Work out the finished part from the listing and answer in its coordinate system (mm). Face numbers are marked on the shaded views. A direction names the side the tool comes from. Round coordinates to 2 decimals unless told otherwise and drop trailing zeros. Write each loop counter-clockwise with the first axis right and the second up, starting at its lowest first coordinate (ties: lowest second). Pieces come first, ordered by that corner, then holes. Notation, with made-up numbers: (10, 52.5) -> (52, 52.5) arc R21 cw to (52, 60.5) -> close; hole circle Ø5 at (53, -33.75). An arc over 180 degrees is marked (long way). Answer as a JSON object with one key per item and string values. Group by question number.
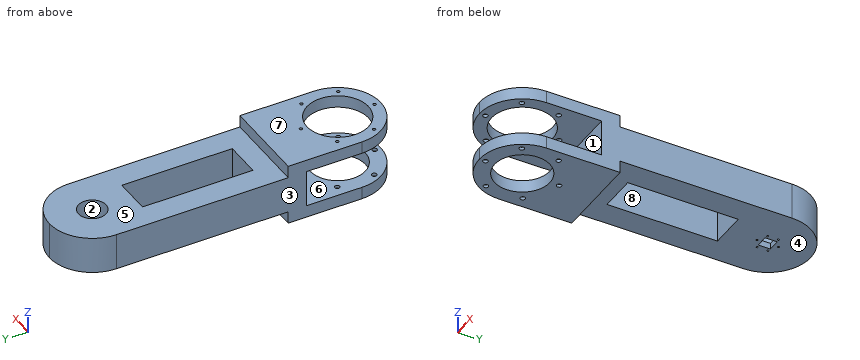
from build123d import *

# Parameters (mm, degrees)
SKETCH_1_W           = 140
SKETCH_1_H           = 350
EXTRUDE_1_DEPTH      = 60
CUT_EXTRUDE_1_REACH  = 199.8
SKETCH_4_W           = 140
SKETCH_4_H           = 100
EXTRUDE_3_DEPTH      = 30
SKETCH_5_W           = 140
SKETCH_5_H           = 20
EXTRUDE_4_DEPTH      = 160
CUT_EXTRUDE_3_DEPTH  = 385.870107959
SKETCH_8_W           = 60
SKETCH_8_H           = 180
CUT_EXTRUDE_4_DEPTH  = 381.164438105
CUT_EXTRUDE_5_REACH  = 386.87
SKETCH_9_R           = 45
CUT_EXTRUDE_6_REACH  = 386.87
SKETCH_10_R          = 50
SKETCH_11_W          = 20
SKETCH_11_H          = 20
CUT_EXTRUDE_7_DEPTH  = 381.164438105
CUT_EXTRUDE_10_REACH = 386.87
SKETCH_13_R          = 2.5
SKETCH_14_R          = 4
CUT_EXTRUDE_11_DEPTH = 5
SKETCH_16_R          = 22.5
SKETCH_16_W          = 20
SKETCH_16_H          = 20
CUT_EXTRUDE_12_DEPTH = 50
SKETCH_17_R          = 1.5
CUT_EXTRUDE_13_DEPTH = 379.186461947
SKETCH_18_R          = 4
CUT_EXTRUDE_14_DEPTH = 5
SKETCH_19_R          = 2.5
CUT_EXTRUDE_15_DEPTH = 385.870107959
CUT_EXTRUDE_START    = -5
SKETCH_20_R          = 4
CUT_EXTRUDE_16_DEPTH = 5


with BuildPart() as part:
    # 草图1 → 凸台-拉伸1 (new body)
    with BuildSketch(Plane.XY):
        Rectangle(SKETCH_1_W, SKETCH_1_H)
    extrude(amount=EXTRUDE_1_DEPTH)

    # 草图2 → 切除-拉伸1 (cut, up to next)
    with BuildSketch(Plane.XY.offset(60), mode=Mode.PRIVATE) as cut_extrude_1_sk1:
        with BuildLine():
            Line((-1.55e-07, 175), (-70, 175))
            Line((-70, 175), (-70, 105))
            ThreePointArc((-70, 105), (-49.497474738, 154.497474628), (-1.55e-07, 175))
        make_face()
    cut_extrude_1_tool1 = extrude(cut_extrude_1_sk1.sketch, amount=-CUT_EXTRUDE_1_REACH, mode=Mode.PRIVATE) & part.part
    # 草图2 → 切除-拉伸1 (cut, up to next)
    with BuildSketch(Plane.XY.offset(60), mode=Mode.PRIVATE) as cut_extrude_1_sk2:
        with BuildLine():
            Line((70, 175), (-1.55e-07, 175))
            ThreePointArc((-1.55e-07, 175), (49.497474628, 154.497474738), (70, 105))
            Line((70, 105), (70, 175))
        make_face()
    cut_extrude_1_tool2 = extrude(cut_extrude_1_sk2.sketch, amount=-CUT_EXTRUDE_1_REACH, mode=Mode.PRIVATE) & part.part
    add(cut_extrude_1_tool1.solids().sort_by_distance((-54.364244, 159.364244, 60))[0], mode=Mode.SUBTRACT)
    add(cut_extrude_1_tool2.solids().sort_by_distance((54.364244, 159.364244, 60))[0], mode=Mode.SUBTRACT)

    # 草图4 → 凸台-拉伸3 (add)
    with BuildSketch(Plane.XZ.offset(175)):
        with Locations((0, 30)):
            Rectangle(SKETCH_4_W, SKETCH_4_H)
    extrude(amount=EXTRUDE_3_DEPTH)

    # 草图5 → 凸台-拉伸4 (add)
    with BuildSketch(Plane.XZ.offset(205)):
        with Locations((0, 70)):
            Rectangle(SKETCH_5_W, SKETCH_5_H)
        with Locations((0, -10)):
            Rectangle(SKETCH_5_W, SKETCH_5_H)
    extrude(amount=EXTRUDE_4_DEPTH)

    # 草图7 → 切除-拉伸3 (cut, through all)
    with BuildSketch(Plane(origin=(0, 0, -20), x_dir=(-1, 0, 0), z_dir=(0, 0, -1))):
        with BuildLine():
            Line((-70, -295), (-70, -365))
            Line((-70, -365), (0, -365))
            ThreePointArc((0, -365), (-49.497474683, -344.497474683), (-70, -295))
        make_face()
        with BuildLine():
            ThreePointArc((70, -295), (49.497474683, -344.497474683), (0, -365))
            Line((0, -365), (70, -365))
            Line((70, -365), (70, -295))
        make_face()
    extrude(amount=-CUT_EXTRUDE_3_DEPTH, mode=Mode.SUBTRACT)

    # 草图8 → 切除-拉伸4 (cut, through all)
    with BuildSketch(Plane(origin=(0, 0, 0), x_dir=(-1, 0, 0), z_dir=(0, 0, -1))):
        with Locations((0, -50)):
            Rectangle(SKETCH_8_W, SKETCH_8_H)
    extrude(amount=-CUT_EXTRUDE_4_DEPTH, mode=Mode.SUBTRACT)

    # 草图9 → 切除-拉伸5 (cut, up to next)
    with BuildSketch(Plane(origin=(0, 0, -20), x_dir=(-1, 0, 0), z_dir=(0, 0, -1)), mode=Mode.PRIVATE) as cut_extrude_5_sk1:
        with Locations((0, -295)):
            Circle(SKETCH_9_R)
    cut_extrude_5_tool1 = extrude(cut_extrude_5_sk1.sketch, amount=-CUT_EXTRUDE_5_REACH, mode=Mode.PRIVATE) & part.part
    add(cut_extrude_5_tool1.solids().sort_by_distance((0, -295, -20))[0], mode=Mode.SUBTRACT)

    # 草图10 → 切除-拉伸6 (cut, up to next)
    with BuildSketch(Plane.XY.offset(80), mode=Mode.PRIVATE) as cut_extrude_6_sk1:
        with Locations((0, -295)):
            Circle(SKETCH_10_R)
    cut_extrude_6_tool1 = extrude(cut_extrude_6_sk1.sketch, amount=-CUT_EXTRUDE_6_REACH, mode=Mode.PRIVATE) & part.part
    add(cut_extrude_6_tool1.solids().sort_by_distance((0, -295, 80))[0], mode=Mode.SUBTRACT)

    # 草图11 → 切除-拉伸7 (cut, through all)
    with BuildSketch(Plane.XY.offset(60)):
        with Locations((0, 105)):
            Rectangle(SKETCH_11_W, SKETCH_11_H)
    extrude(amount=-CUT_EXTRUDE_7_DEPTH, mode=Mode.SUBTRACT)

    # 草图13 → 切除-拉伸10 (cut, up to next)
    with BuildSketch(Plane.XY.offset(80), mode=Mode.PRIVATE) as cut_extrude_10_sk1:
        with Locations((-51.961524227, -265)):
            Circle(SKETCH_13_R)
    cut_extrude_10_tool1 = extrude(cut_extrude_10_sk1.sketch, amount=-CUT_EXTRUDE_10_REACH, mode=Mode.PRIVATE) & part.part
    # 草图13 → 切除-拉伸10 (cut, up to next)
    with BuildSketch(Plane.XY.offset(80), mode=Mode.PRIVATE) as cut_extrude_10_sk2:
        with Locations((0, -235)):
            Circle(SKETCH_13_R)
    cut_extrude_10_tool2 = extrude(cut_extrude_10_sk2.sketch, amount=-CUT_EXTRUDE_10_REACH, mode=Mode.PRIVATE) & part.part
    # 草图13 → 切除-拉伸10 (cut, up to next)
    with BuildSketch(Plane.XY.offset(80), mode=Mode.PRIVATE) as cut_extrude_10_sk3:
        with Locations((51.961524227, -265)):
            Circle(SKETCH_13_R)
    cut_extrude_10_tool3 = extrude(cut_extrude_10_sk3.sketch, amount=-CUT_EXTRUDE_10_REACH, mode=Mode.PRIVATE) & part.part
    # 草图13 → 切除-拉伸10 (cut, up to next)
    with BuildSketch(Plane.XY.offset(80), mode=Mode.PRIVATE) as cut_extrude_10_sk4:
        with Locations((51.961524227, -325)):
            Circle(SKETCH_13_R)
    cut_extrude_10_tool4 = extrude(cut_extrude_10_sk4.sketch, amount=-CUT_EXTRUDE_10_REACH, mode=Mode.PRIVATE) & part.part
    # 草图13 → 切除-拉伸10 (cut, up to next)
    with BuildSketch(Plane.XY.offset(80), mode=Mode.PRIVATE) as cut_extrude_10_sk5:
        with Locations((0, -355)):
            Circle(SKETCH_13_R)
    cut_extrude_10_tool5 = extrude(cut_extrude_10_sk5.sketch, amount=-CUT_EXTRUDE_10_REACH, mode=Mode.PRIVATE) & part.part
    # 草图13 → 切除-拉伸10 (cut, up to next)
    with BuildSketch(Plane.XY.offset(80), mode=Mode.PRIVATE) as cut_extrude_10_sk6:
        with Locations((-51.961524227, -325)):
            Circle(SKETCH_13_R)
    cut_extrude_10_tool6 = extrude(cut_extrude_10_sk6.sketch, amount=-CUT_EXTRUDE_10_REACH, mode=Mode.PRIVATE) & part.part
    add(cut_extrude_10_tool1.solids().sort_by_distance((-51.961524, -265, 80))[0], mode=Mode.SUBTRACT)
    add(cut_extrude_10_tool2.solids().sort_by_distance((0, -235, 80))[0], mode=Mode.SUBTRACT)
    add(cut_extrude_10_tool3.solids().sort_by_distance((51.961524, -265, 80))[0], mode=Mode.SUBTRACT)
    add(cut_extrude_10_tool4.solids().sort_by_distance((51.961524, -325, 80))[0], mode=Mode.SUBTRACT)
    add(cut_extrude_10_tool5.solids().sort_by_distance((0, -355, 80))[0], mode=Mode.SUBTRACT)
    add(cut_extrude_10_tool6.solids().sort_by_distance((-51.961524, -325, 80))[0], mode=Mode.SUBTRACT)

    # 草图14 → 切除-拉伸11 (cut)
    with BuildSketch(Plane(origin=(0, 0, 60), x_dir=(-1, 0, 0), z_dir=(0, 0, -1))):
        with Locations((-51.961524227, -325)):
            Circle(SKETCH_14_R)
        with Locations((-51.961524227, -265)):
            Circle(SKETCH_14_R)
        with Locations((0, -235)):
            Circle(SKETCH_14_R)
        with Locations((51.961524227, -265)):
            Circle(SKETCH_14_R)
        with Locations((51.961524227, -325)):
            Circle(SKETCH_14_R)
        with Locations((0, -355)):
            Circle(SKETCH_14_R)
    extrude(amount=-CUT_EXTRUDE_11_DEPTH, mode=Mode.SUBTRACT)

    # 草图16 → 切除-拉伸12 (cut)
    with BuildSketch(Plane.XY.offset(60)):
        with Locations((0, 105)):
            Circle(SKETCH_16_R)
        with Locations((0, 105)):
            Rectangle(SKETCH_16_W, SKETCH_16_H, mode=Mode.SUBTRACT)
    extrude(amount=-CUT_EXTRUDE_12_DEPTH, mode=Mode.SUBTRACT)

    # 草图17 → 切除-拉伸13 (cut, through all)
    with BuildSketch(Plane.XY.offset(10)):
        with Locations((0, 122.5)):
            Circle(SKETCH_17_R)
        with Locations((15.155444566, 113.75)):
            Circle(SKETCH_17_R)
        with Locations((15.155444566, 96.25)):
            Circle(SKETCH_17_R)
        with Locations((0, 87.5)):
            Circle(SKETCH_17_R)
        with Locations((-15.155444566, 96.25)):
            Circle(SKETCH_17_R)
        with Locations((-15.155444566, 113.75)):
            Circle(SKETCH_17_R)
    extrude(amount=-CUT_EXTRUDE_13_DEPTH, mode=Mode.SUBTRACT)

    # 草图18 → 切除-拉伸14 (cut)
    with BuildSketch(Plane(origin=(0, 0, -20), x_dir=(-1, 0, 0), z_dir=(0, 0, -1))):
        with Locations((0, -235)):
            Circle(SKETCH_18_R)
        with Locations((-51.961524227, -265)):
            Circle(SKETCH_18_R)
        with Locations((-51.961524227, -325)):
            Circle(SKETCH_18_R)
        with Locations((0, -355)):
            Circle(SKETCH_18_R)
        with Locations((51.961524227, -325)):
            Circle(SKETCH_18_R)
        with Locations((51.961524227, -265)):
            Circle(SKETCH_18_R)
    extrude(amount=-CUT_EXTRUDE_14_DEPTH, mode=Mode.SUBTRACT)

    # 草图19 → 切除-拉伸15 (cut, through all)
    with BuildSketch(Plane(origin=(0, 0, -20), x_dir=(-1, 0, 0), z_dir=(0, 0, -1))):
        with Locations(Location((-51.961524227, -265, 0), (0, 0, 180))):
            Circle(SKETCH_19_R)
        with Locations(Location((-51.961524227, -325, 0), (0, 0, 180))):
            Circle(SKETCH_19_R)
        with Locations(Location((0, -355, 0), (0, 0, 180))):
            Circle(SKETCH_19_R)
        with Locations(Location((51.961524227, -325, 0), (0, 0, 180))):
            Circle(SKETCH_19_R)
        with Locations(Location((51.961524227, -265, 0), (0, 0, 180))):
            Circle(SKETCH_19_R)
        with Locations(Location((0, -235, 0), (0, 0, 180))):
            Circle(SKETCH_19_R)
    extrude(amount=-CUT_EXTRUDE_15_DEPTH, mode=Mode.SUBTRACT)

    # 草图20 → 切除-拉伸16 (cut)
    with BuildSketch(Plane.XY.offset(CUT_EXTRUDE_START)):
        with Locations(Location((-51.961524227, -265, 0), (0, 0, 180))):
            Circle(SKETCH_20_R)
        with Locations((0.040572827, -234.996244649)):
            Circle(SKETCH_20_R)
        with Locations((52.025635698, -265.029504072)):
            Circle(SKETCH_20_R)
        with Locations((52.008601514, -325.066518847)):
            Circle(SKETCH_20_R)
        with Locations((0.00650446, -355.070274198)):
            Circle(SKETCH_20_R)
        with Locations((-51.978558411, -325.037014775)):
            Circle(SKETCH_20_R)
    extrude(amount=CUT_EXTRUDE_16_DEPTH, mode=Mode.SUBTRACT)


solid = part.part
1) A tool of negligible diameter and unlimited length cuts with its end or side. For the marked faces 4, 5, 6, 7 and 8, from which of +Z, -Z, +X, -X, +Y, -Y can it reach the whole face along a straight path? Write none if from no direction.
2) For a pull along X with two mould halves and no side action, classify the marked faces 1, 2 and 3 as released by +X, released by -X, zero draft, split by the parting line, or undercut.
3) A cutting plane is placed at C-C on x = 39. Determine the outline of the cut face in (y, z), plus the area to 3 significant figures.
4) A cutting plane is placed at B-B on z = 40.5. Determine the outline of the cut face in (x, y), plus the area to 3 significant figures.
5) Each of these flat-tipped pins is pushed along its axis until it touches: P1, Ø2.5, axis at x = -53.5, y = -265.5, coming from the -Z side; P2, Ø3, axis at x = 51.96, y = -325, coming from the -Z side; P3, Ø2, axis at x = 21, z = 3, coming from the +Y side; P4, Ø1, axis at x = -21.5, y = -166.5, coming from the -Z side. Where does it stop, or does it pass through?
6) A cutting plane is placed at A-A on y = -135. Determine the outline of the cut face in (x, z), plus the area to 3 significant figures.
7) Straight lines are drawn through the part: L1, parallel to X at y = 31.5, z = 21.5; L2, parallel to Y at x = 51.5, z = 76.5; L3, parallel to Z at x = -58.5, y = -301. For each, find the intervals that lie inside material, in ascending order.
Established:
{
 "1": {"face 4": "-Z, +X, -X, +Y", "face 5": "+Z, +X, -X, +Y", "face 6": "+X, -X, -Y", "face 7": "+Z, +X, -X, +Y, -Y", "face 8": "+Z, -Z"},
 "2": {"face 1": "zero draft", "face 2": "undercut", "face 3": "released by -X"},
 "3": {"outline": "(-353.13, -20) -> (-317.45, -20) -> (-317.45, 0) -> (-353.13, 0) -> close; (-353.13, 60) -> (-326.29, 60) -> (-326.29, 80) -> (-353.13, 80) -> close; (-272.55, -20) -> (-175, -20) -> (-175, 0) -> (163.13, 0) -> (163.13, 60) -> (-175, 60) -> (-175, 80) -> (-263.71, 80) -> (-263.71, 60) -> (-205, 60) -> (-205, 0) -> (-272.55, 0) -> close", "area": "27,100 mm²"},
 "4": {"outline": "(-70, -205) -> (70, -205) -> (70, 105) arc R70 ccw to (-70, 105) -> close; hole (-30, -140) -> (30, -140) -> (30, 40) -> (-30, 40) -> close; hole circle Ø45 at (0, 105)", "area": "38,700 mm²"},
 "5": {"P1": "stops at z = -15", "P2": "passes through", "P3": "stops at y = 172.08", "P4": "stops at z = 0"},
 "6": {"outline": "(-70, 0) -> (-30, 0) -> (-30, 60) -> (-70, 60) -> close; (30, 0) -> (70, 0) -> (70, 60) -> (30, 60) -> close", "area": "4,800 mm²"},
 "7": {"L1": "x = -70 to -30, 30 to 70", "L2": "y = -342.41 to -327.46, -322.54 to -267.46, -262.54 to -175", "L3": "z = -20 to 0, 60 to 80"}
}
